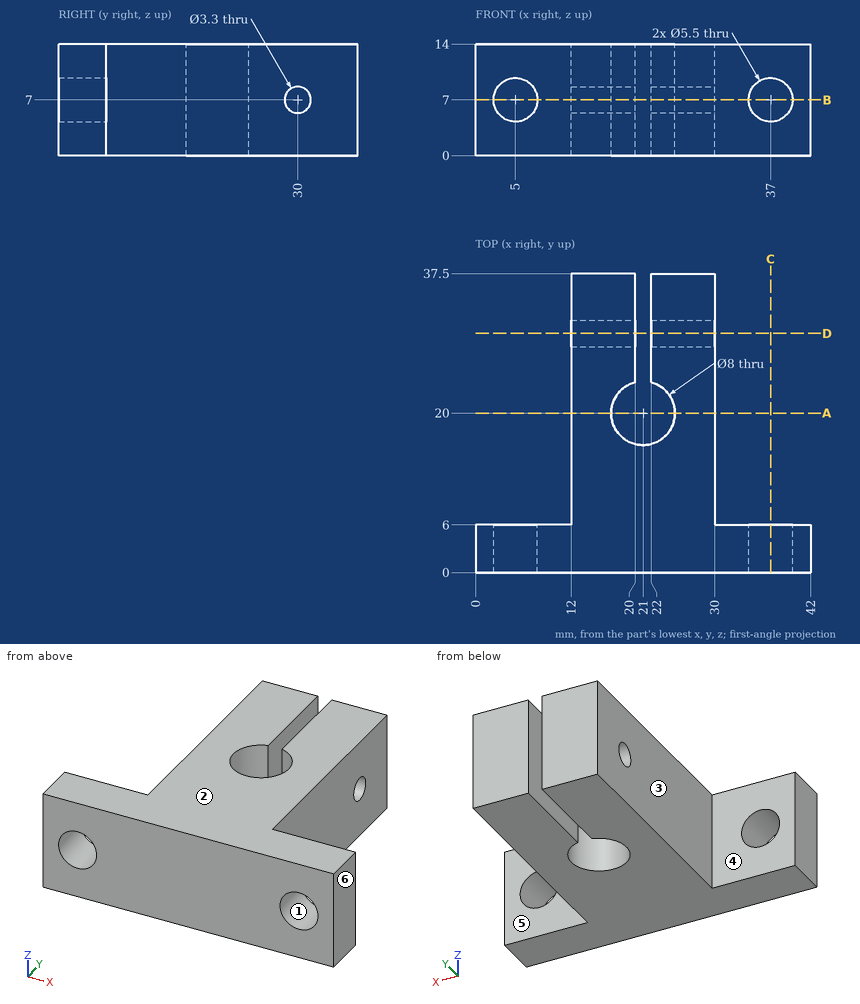
Geometry: see drawing. Coordinates: mm, zero at the bounding-box minimum. A direction names the side the tool comes from. Coordinates: 2 decimals unless noted, no trailing zeros. Loops run counter-clockwise (first coordinate to the right, second up) from the corner with the lowest first, then second, coordinate; pieces in that order, holes last. Notation, with made-up numbers: (58.5, 37.25) - (85.5, 37.25) arc R15 cw to (85.5, 51.25) - close; hole circle Ø8 at (53.5, -9). An arc over 180 degrees is marked (long way). Return JSON: item names as keys, results as strings.
Q1. Access query for the marked faces 4, 5 and 6. Directions: +Z, -Z, +X, -X, +Y, -Y. A direction counts if a zero-diameter tool reaches every point of the face in a straight line with its end or side. Return the directions, or none.
Results:
{"face 4": "+Z, -Z, -X, +Y", "face 5": "+Z, -Z, +X, +Y", "face 6": "+Z, -Z, +X, +Y, -Y"}
Q2. Section C-C, the plane x = 37. Return loops of the section in (y, z), plus the area to 3 significant figures.
Results:
{"outline": "(0, 0) - (6, 0) - (6, 4.25) - (0, 4.25) - close; (0, 9.75) - (6, 9.75) - (6, 14) - (0, 14) - close", "area": "51.0 mm2"}
Q3. Section D-D, the plane y = 30. Return loops of the section in (x, z), plus the area to 3 significant figures.
Results:
{"outline": "(12, 0) - (20, 0) - (20, 5.35) - (12, 5.35) - close; (12, 8.65) - (20, 8.65) - (20, 14) - (12, 14) - close; (22, 0) - (30, 0) - (30, 5.35) - (22, 5.35) - close; (22, 8.65) - (30, 8.65) - (30, 14) - (22, 14) - close", "area": "171 mm2"}
Q4. Section A-A, the plane y = 20. Return loops of the section in (x, z), plus the area to 3 significant figures.
Results:
{"outline": "(12, 0) - (17, 0) - (17, 14) - (12, 14) - close; (25, 0) - (30, 0) - (30, 14) - (25, 14) - close", "area": "140 mm2"}
Q5. Contact query for flat-ended pins moving along their axis: P1, Ø7, axis at y = 23.5, z = 9.5, coming from the -X side; P2, Ø4, axis at y = 18.5, z = 11, coming from the +X side. Output: stop coordinate, or through.
Results:
{"P1": "x = 12", "P2": "x = 30"}
Q6. Mould query, pull axis Z, two halves, no side actions, for the marked faces 1, 2 and 3. Classes: released by +Z, released by -Z, zero draft, split by the parting line, or undercut.
Results:
{"face 1": "undercut", "face 2": "released by +Z", "face 3": "zero draft"}
Q7. Section B-B, the plane z = 7. Return loops of the section in (x, y), plus the area to 3 significant figures.
Results:
{"outline": "(0, 0) - (2.25, 0) - (2.25, 6) - (0, 6) - close; (7.75, 0) - (34.25, 0) - (34.25, 6) - (30, 6) - (30, 28.35) - (22, 28.35) - (22, 23.87) arc R4 cw (long way) to (20, 23.87) - (20, 28.35) - (12, 28.35) - (12, 6) - (7.75, 6) - close; (12, 31.65) - (20, 31.65) - (20, 37.5) - (12, 37.5) - close; (22, 31.65) - (30, 31.65) - (30, 37.5) - (22, 37.5) - close; (39.75, 0) - (42, 0) - (42, 6) - (39.75, 6) - close", "area": "623 mm2"}
Q8. Material intervals for line 1 along X through (y, z) = (27, 2.25); line 2 along X through (y, z) = (20, 3); line 3 along Z through (x, y) = (37, 2.75), sorted ascending.
Results:
{"line 1": "12 to 20, 22 to 30", "line 2": "12 to 17, 25 to 30", "line 3": "0 to 4.25, 9.75 to 14"}
